Verification items for the finished model (mm, model axes). Round coordinates to 2 decimals unless told otherwise and drop trailing zeros. Order: outer loops, then holes, each group sorted by start corner. A loop starts at its lowest first (then second) coordinate and runs counter-clockwise, first axis right, second up. Notation, with made-up numbers: (-4.75, 40.25) -> (25.25, 40.25) arc R17 cw to (25.25, 61.25) -> close; hole circle Ø8 at (3, 7). An arc over 180 degrees is marked (long way). Return JSON: item names as keys, results as strings. Group by question number.
Item 1: Scan lines: probe 1 along X at (y, z) = (0, 8.8); probe 2 along X at (y, z) = (0, 4.5); probe 3 along Y at (x, z) = (17, 8.1). Record each from-to range of solid material in increasing order. Write a range as from..to.
Item 2: Depth check by flat-ended pin: pin 1 Ø1.9 at (x, y) = (-17, 0) entering from +Z; pin 2 Ø3.5 at (x, y) = (17, 0) entering from +Z. Enter the tip coordinate at first touch or a pass-through.
Item 3: Sectioned sample at C-C on z = 5.5. Record the cut outline in (x, y), plus the area to 3 significant figures.
Item 4: Sectioned sample at A-A on y = 0. Record the cut outline in (x, z), plus the area to 3 significant figures.
Item 5: Sectioned sample at B-B on x = -17. Record the cut outline in (y, z), plus the area to 3 significant figures.
Item 6: Sectioned sample at D-D on x = 17.5. Record the cut outline in (y, z).
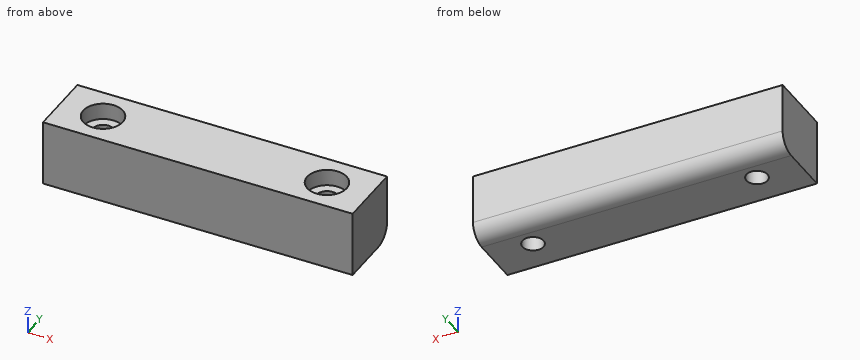
Autodesk Inventor part; units mm, degrees
ref_plane "YZ Plane" through (0, 0, 0) normal (1, 0, 0) x (0, 1, 0)
ref_plane "XZ Plane" through (0, 0, 0) normal (0, 1, 0) x (-1, 0, 0)
ref_plane "XY Plane" through (0, 0, 0) normal (0, 0, 1) x (1, 0, 0)
sketch "Sketch1" plane through (0, 0, 0) normal (0, 0, 1) x (1, 0, 0)
  line L0 (-23.5, -5) -> (23.5, -5)
  line L1 (23.5, -5) -> (23.5, 5)
  line L2 (23.5, 5) -> (-23.5, 5)
  line L3 (-23.5, 5) -> (-23.5, -5)
  line L4 (-23.5, -5) -> (23.5, 5) construction
  line L5 (23.5, -5) -> (-23.5, 5) construction
  point P0 (0, 0)
  dimension "d0" = 47
  dimension "d1" = 10
extrude "Extrusion1" add sketch "Sketch1" along normal blind 10
sketch "Sketch2" plane through (0, 0, 10) normal (0, 0, 1) x (1, 0, 0)
  line L0 (-23.5, 5) -> (-23.5, -5)
  line L1 (-23.5, 0) -> (-17, 0)
  line L2 (-17, 0) -> (17, 0)
  point P0 (0, 0)
  dimension "d4" = 6.5
  dimension "d5" = 34
hole "Hole1" at (-17, 0, 10) at (17, 0, 10) direction (0, 0, -1) diameter 3.2 end through all counterbore diameter 6 counterbore depth 2.5
fillet "Fillet1" radius 2.5 1 edges at (0, 5, 0)
properties part number "Satupofa"
Recorded:
{
 "1": {"probe 1": "-23.5..-20, -14..14, 20..23.5", "probe 2": "-23.5..-18.6, -15.4..15.4, 18.6..23.5", "probe 3": "-5..-3, 3..5"},
 "2": {"pin 1": "through", "pin 2": "z = 7.5"},
 "3": {"outline": "(-23.5, -5) -> (23.5, -5) -> (23.5, 5) -> (-23.5, 5) -> close; hole circle Ø3.2 at (-17, 0); hole circle Ø3.2 at (17, 0)", "area": "454 mm²"},
 "4": {"outline": "(-23.5, 0) -> (-18.6, 0) -> (-18.6, 7.5) -> (-20, 7.5) -> (-20, 10) -> (-23.5, 10) -> close; (-15.4, 0) -> (15.4, 0) -> (15.4, 7.5) -> (14, 7.5) -> (14, 10) -> (-14, 10) -> (-14, 7.5) -> (-15.4, 7.5) -> close; (18.6, 0) -> (23.5, 0) -> (23.5, 10) -> (20, 10) -> (20, 7.5) -> (18.6, 7.5) -> close", "area": "392 mm²"},
 "5": {"outline": "(-5, 0) -> (-1.6, 0) -> (-1.6, 7.5) -> (-3, 7.5) -> (-3, 10) -> (-5, 10) -> close; (1.6, 0) -> (2.5, 0) arc R2.5 ccw to (5, 2.5) -> (5, 10) -> (3, 10) -> (3, 7.5) -> (1.6, 7.5) -> close", "area": "59.7 mm²"},
 "6": {"outline": "(-5, 0) -> (-1.52, 0) -> (-1.52, 7.5) -> (-2.96, 7.5) -> (-2.96, 10) -> (-5, 10) -> close; (1.52, 0) -> (2.5, 0) arc R2.5 ccw to (5, 2.5) -> (5, 10) -> (2.96, 10) -> (2.96, 7.5) -> (1.52, 7.5) -> close"}
}
